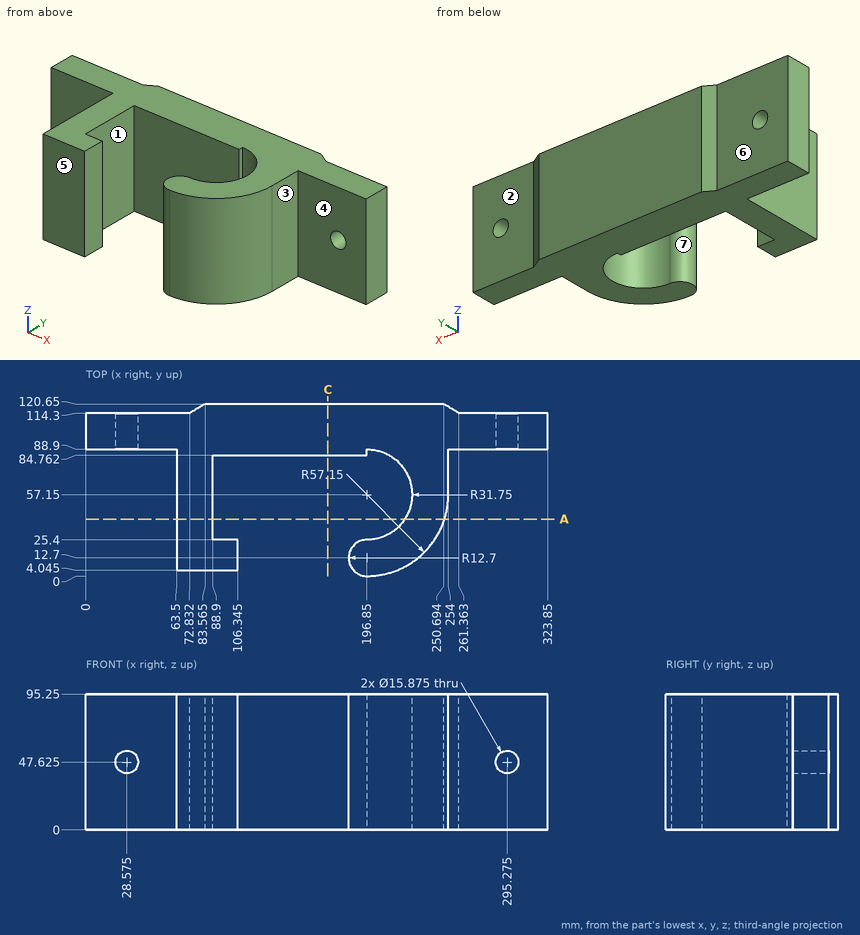
Input: dimensioned drawing with shaded views. Units: mm. Origin: part minimum x, y, z. A direction names the side the tool comes from. Round coordinates to 2 decimals unless told otherwise and drop trailing zeros. Loops run counter-clockwise (first coordinate to the right, second up) from the corner with the lowest first, then second, coordinate; pieces in that order, holes last. Notation, with made-up numbers: (-3, 31) -> (21, 31) arc R30 ccw to (21, 64) -> close; hole circle Ø1 at (48, -31.75). An arc over 180 degrees is marked (long way). Answer as a JSON object with one key per item and string values. Group by question number.
Q1. Access query for the marked faces 4, 5, 6 and 7. Directions: +Z, -Z, +X, -X, +Y, -Y. A direction counts if a zero-diameter tool reaches every point of the face in a straight line with its end or side. Return the directions, or none.
Q2. Contact query for flat-ended pins moving along their axis: P1, Ø3.5, axis at y = 86.5, z = 32.5, coming from the +X side; P2, Ø12, axis at x = 257, z = 51, coming from the +Y side; P3, Ø1, axis at y = 72.5, z = 68, coming from the -X side. Output: stop coordinate, or through.
Q3. Ray query, line 1 (Y direction, x = 17.5, z = 86); line 2 (Y direction, x = 153.5, z = 4.5); line 3 (X direction, y = 83.5, z = 8.5) (1 decimal). Return the intervals inside material, ascending. Write a range as from..to.
Q4. Mould query, pull axis X, two halves, no side actions, for the marked faces 1, 2 and 3. Classes: pulls with the +X half, pulls with the -X half, needs draft (parallel to the pull), parting line crosses it, or undercut.
Q5. Section query A-A (y = 40). Output: boundary loops of the cut face in (x, z).
Q6. Section query C-C (x = 169.5). Output: boundary loops of the cut face in (y, z), plus the area to 3 significant figures.
Completed:
{
 "1": {"face 4": "+Z, -Z, +X, -Y", "face 5": "+Z, -Z, -X, -Y", "face 6": "+Z, -Z, -X, +Y", "face 7": "+Z, -Z"},
 "2": {"P1": "x = 254", "P2": "y = 120.47", "P3": "x = 63.5"},
 "3": {"line 1": "88.9..114.3", "line 2": "84.76..120.65", "line 3": "63.5..88.9, 214.6..254"},
 "4": {"face 1": "undercut", "face 2": "needs draft", "face 3": "pulls with the +X half"},
 "5": {"outline": "(63.5, 0) -> (88.9, 0) -> (88.9, 95.25) -> (63.5, 95.25) -> close; (223.57, 0) -> (251.37, 0) -> (251.37, 95.25) -> (223.57, 95.25) -> close"},
 "6": {"outline": "(84.76, 0) -> (120.65, 0) -> (120.65, 95.25) -> (84.76, 95.25) -> close", "area": "3,420 mm²"}
}
